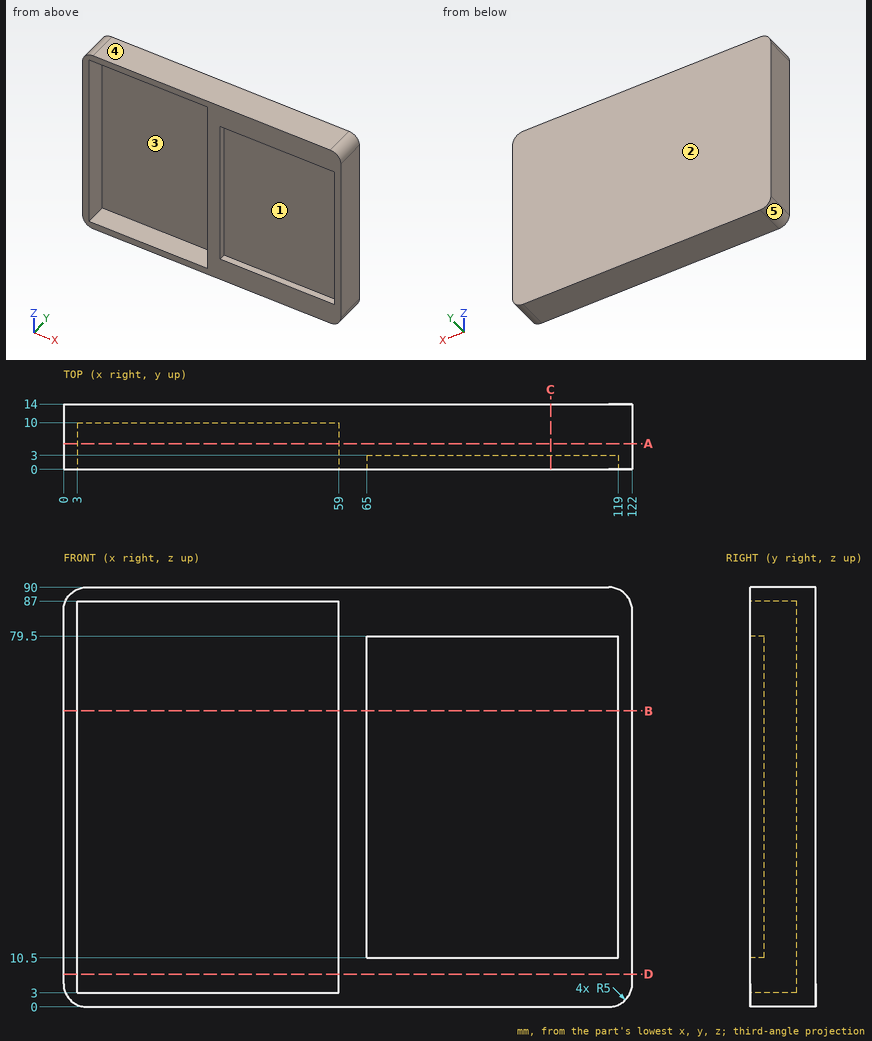
Design review of the part shown in the three views and the two pictorial views. Dimensions are in mm from the part's minimum x, y and z. A direction names the side the tool comes from. Round coordinates to 2 decimals unless told otherwise and drop trailing zeros. Write each loop counter-clockwise with the first axis right and the second up, starting at its lowest first coordinate (ties: lowest second). Pieces come first, ordered by that corner, then holes.
Item 1: Consider section C-C on x = 104.5. Give the boundary of the cut face in (y, z).
Item 2: Draft analysis for pull direction X (two halves, no side actions). For the marked faces 3, 4 and 5, state which applies: released by +X, released by -X, zero draft, split by the parting line, or undercut.
Item 3: Wall thickness on L1, parallel to X at y = 3, z = 6; L2, parallel to Z at x = 56, y = 4.25; L3, parallel to Z at x = 81.5, y = 1.5: over which ranges is each line inside the solid? List them lowest first.
Item 4: For the marked faces 1 and 2, list the 3-axis set-ups (+Z, -Z, +X, -X, +Y, -Y) from which the entire face can be reached by the end or side of a thin tool; tool diameter is ignored.
Item 5: Consider section D-D on z = 7. Give the boundary of the cut face in (x, y).
Item 6: Consider section B-B on z = 63.5. Give the boundary of the cut face in (x, y).
Item 7: Consider section A-A on y = 5.5. Give the boundary of the cut face in (x, z), and give its area (3 significant figures).
Item 8: For pin 1 Ø5 at (y, z) = (3.5, 49) entering from -X, flat-tipped, find the tip position at first contact; note if it passes through.
Check values:
1. outline: (0, 0) - (14, 0) - (14, 90) - (0, 90) - (0, 79.5) - (3, 79.5) - (3, 10.5) - (0, 10.5) - close
2. face 3: undercut
2. face 4: zero draft
2. face 5: released by -X
3. L1: x = 0 to 3, 59 to 122
3. L2: z = 0 to 3, 87 to 90
3. L3: z = 0 to 10.5, 79.5 to 90
4. face 1: -Y
4. face 2: +Z, -Z, +X, -X, +Y
5. outline: (0, 0) - (3, 0) - (3, 10) - (59, 10) - (59, 0) - (122, 0) - (122, 14) - (0, 14) - close
6. outline: (0, 0) - (3, 0) - (3, 10) - (59, 10) - (59, 0) - (65, 0) - (65, 3) - (119, 3) - (119, 0) - (122, 0) - (122, 14) - (0, 14) - close
7. outline: (0, 5) arc R5 ccw to (5, 0) - (117, 0) arc R5 ccw to (122, 5) - (122, 85) arc R5 ccw to (117, 90) - (5, 90) arc R5 ccw to (0, 85) - close; hole (3, 3) - (59, 3) - (59, 87) - (3, 87) - close
7. area: 6,250 mm2
8. pin 1: stops at x = 0
